from build123d import *

# Parameters (mm, degrees)
ELEC_CH_SKETCH_W         = 0.2
ELEC_CH_SKETCH_H         = 2
SKETCH2_R                = 0.18
BOSS_EXTRUDE1_DEPTH      = 19
BOSS_EXTRUDE1_DEPTH_BACK = 8
SKETCH3_W                = 5
SKETCH3_H                = 8
SKETCH5_W                = 14
SKETCH5_H                = 2
CUT_EXTRUDE1_DEPTH       = 3.5


with BuildPart() as part:
    # Sweep2: sweep along a path in guide
    with BuildLine(Plane(origin=(0, 0, 0), x_dir=(-1, 0, 0), z_dir=(0, 1, 0))) as sweep2_path:
        Line((0, 0), (-15, 0))
    # elec_ch_sketch → Sweep2 (sweep)
    with BuildSketch(Plane.YZ):
        Rectangle(ELEC_CH_SKETCH_W, ELEC_CH_SKETCH_H)
    sweep(path=sweep2_path.line)



with BuildPart() as body_2:
    # Sweep3: sweep along a path in guide<3>
    with BuildLine(Plane(origin=(0, 0, 0), x_dir=(-1, 0, 0), z_dir=(0, 1, 0))) as sweep3_path:
        Line((4, 0), (6, 0))
        ThreePointArc((6, 0), (7.414213562, 0.585786438), (8, 2))
    # Sketch2 → Sweep3 (sweep)
    with BuildSketch(Plane(origin=(-4, 0, 0), x_dir=(0, 0, -1), z_dir=(1, 0, 0))):
        Circle(SKETCH2_R)
    sweep(path=sweep3_path.line)


with BuildPart() as part_1:
    add(part.part)

    add(body_2.part)  # Loft1 merges body 2
    # Sketch2<3> for Loft1 → Loft1 section 0
    with BuildSketch(Plane(origin=(-4, 0, 0), x_dir=(0, 0, -1), z_dir=(1, 0, 0))):
        with BuildLine():
            # circular arc as an exact rational Bezier (weights 1, cos(half-angle), 1)
            Bezier((0.179106694, -0.017910669), (0.180897761, 0), (0.179106694, 0.017910669), weights=[1, 0.995037187, 1])
            Bezier((0.179106694, 0.017910669), (0, 1.80897768), (-0.179106694, 0.017910669), weights=[1, 0.099503715, 1])
            Bezier((-0.179106694, 0.017910669), (-0.180897761, 0), (-0.179106694, -0.017910669), weights=[1, 0.995037187, 1])
            Bezier((-0.179106694, -0.017910669), (0, -1.80897768), (0.179106694, -0.017910669), weights=[1, 0.099503715, 1])
        make_face()
    # elec_ch_sketch<3> → Loft1 section 1
    with BuildSketch(Plane.YZ):
        with BuildLine():
            Line((-0.1, -1), (0.1, -1))
            Line((0.1, -1), (0.1, 1))
            Line((0.1, 1), (-0.1, 1))
            Line((-0.1, 1), (-0.1, -1))
        make_face()
    loft()


with BuildPart() as body_2_2:
    # Sketch3 → Boss-Extrude1 (new, two sides: drawn at the far end of the back side and taken through both)
    with BuildSketch(Plane(origin=(-4, 0, 0), x_dir=(0, 0, -1), z_dir=(1, 0, 0)).offset(-BOSS_EXTRUDE1_DEPTH_BACK)):
        with Locations((0.5, 0)):
            Rectangle(SKETCH3_W, SKETCH3_H)
    extrude(amount=BOSS_EXTRUDE1_DEPTH + BOSS_EXTRUDE1_DEPTH_BACK)

    # Combine1: cut part
    add(part_1.part, mode=Mode.SUBTRACT)

    # Sketch5 → Cut-Extrude1 (cut)
    with BuildSketch(Plane.XY.offset(2)):
        with Locations((8, -1.2)):
            Rectangle(SKETCH5_W, SKETCH5_H)
        with Locations((8, 1.2)):
            Rectangle(SKETCH5_W, SKETCH5_H)
    extrude(amount=-CUT_EXTRUDE1_DEPTH, mode=Mode.SUBTRACT)


solid = body_2_2.part
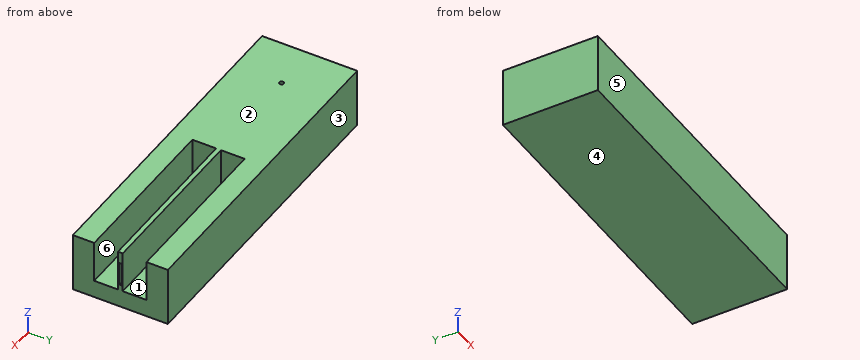
Source: CAD feature listing. Evaluate the final solid. Frame: model axes, mm. Face numbers are marked on the shaded views. A direction names the side the tool comes from. Give positions to 0.01 mm unless a question says otherwise; leave off trailing zeros. Loops run counter-clockwise (first coordinate to the right, second up) from the corner with the lowest first, then second, coordinate; pieces in that order, holes last. Notation, with made-up numbers: (37.5, -27.75) -> (81.5, -27.75) arc R15 ccw to (81.5, -6.75) -> close; hole circle Ø10 at (89.25, -14). An arc over 180 degrees is marked (long way). Use a Markdown table: item, result. Add a question column.
1) First-contact query: pin 1 (0.6 mm diameter, centred on y = 1.5, z = 0.5, fed in from +X); pin 2 (1 mm diameter, centred on x = 6, y = -1, fed in from +Z); pin 3 (2 mm diameter, centred on x = 7, y = 1, fed in from +Z). Flat tips, straight axial feed; report the tip coordinate or a pass-through.
2) Reachability of the marked faces 1 and 2 from +Z, -Z, +X, -X, +Y, -Y: full face, straight path, thin tool, end or side. Return the list, or none.
3) Pull-direction query (Y, two-part tool) for the marked faces 3, 4, 5 and 6; classes: +Y half, -Y half, draft (parallel to the pull), parting line (faces both ways), or undercut.
4) Line query: line 1 along Y through (x, z) = (2, -1.2); line 2 along Z through (x, y) = (-4.95, 0); line 3 along Y through (x, z) = (-4.8, 0). Output: solid intervals per line, ascending. Write a range as [from, to].
5) Section query B-B, the plane y = 1.75. Return the cut outline in (x, z), then the cut area to 3 significant figures.
6) Section query A-A, the plane x = 4.25. Return the cut outline in (y, z), then the cut area to 3 significant figures.
Numbers:
| question | item | result |
|---|---|---|
| 1 | pin 1 | stops at x = 1 |
| 1 | pin 2 | stops at z = -1.5 |
| 1 | pin 3 | stops at z = 2 |
| 2 | face 1 | +Z, +X |
| 2 | face 2 | +Z, +X, -X, +Y, -Y |
| 3 | face 3 | +Y half |
| 3 | face 4 | draft |
| 3 | face 5 | -Y half |
| 3 | face 6 | undercut |
| 4 | line 1 | y = [-4, -2.2], [-0.2, 0.2], [2.2, 4] |
| 4 | line 2 | z = [-3, -0.18], [0.18, 2] |
| 4 | line 3 | y = [-4, -0.18], [0.18, 4] |
| 5 | outline | (-12, -3) -> (15, -3) -> (15, -1.5) -> (1, -1.5) -> (1, 2) -> (-12, 2) -> close |
| 5 | area | 86.0 mm2 |
| 6 | outline | (-4, -3) -> (4, -3) -> (4, 2) -> (2.2, 2) -> (2.2, -1.5) -> (0.2, -1.5) -> (0.2, 2) -> (-0.2, 2) -> (-0.2, -1.5) -> (-2.2, -1.5) -> (-2.2, 2) -> (-4, 2) -> close; hole (-0.1, -1) -> (0.1, -1) -> (0.1, 1) -> (-0.1, 1) -> close |
| 6 | area | 25.6 mm2 |
